```python
from build123d import *

# Parameters (mm, degrees)
AUFSATZ_LINEAR_AUSTRAGEN1_DEPTH    = 5
F_4_0_4_DURCHMESSER_BOHRUNG1_D     = 4
F_4_0_4_DURCHMESSER_BOHRUNG1_DEPTH = 5
F_4_0_4_DURCHMESSER_BOHRUNG1_TIP   = 1.201721238


with BuildPart() as part:
    # Skizze2 → Aufsatz-Linear austragen1 (new body)
    with BuildSketch(Plane.XY):
        with BuildLine():
            Line((1.443375673, 0), (38.556624327, 0))
            ThreePointArc((38.556624327, 0), (39.806624327, -0.334936491), (40.721687836, -1.25))
            Line((40.721687836, -1.25), (50.680145631, -18.498554865))
            ThreePointArc((50.680145631, -18.498554865), (52.51027265, -20.328681884), (55.01027265, -20.998554865))
            Line((55.01027265, -20.998554865), (62.123521304, -20.998554865))
            ThreePointArc((62.123521304, -20.998554865), (64.623521304, -22.034088771), (67.123521304, -20.998554865))
            Line((67.123521304, -20.998554865), (74.793302349, -20.998554865))
            ThreePointArc((74.793302349, -20.998554865), (76.005598743, -20.827762698), (77.123521304, -20.328681884))
            Line((77.123521304, -20.328681884), (77.123521304, -32.998554865))
            ThreePointArc((77.123521304, -32.998554865), (20.139660848, -90.963323142), (-37.5, -33.650635095))
            Line((-37.5, -33.650635095), (-37.501029815, -20.980635095))
            ThreePointArc((-37.501029815, -20.980635095), (-36.382703591, -21.479811555), (-35.17, -21.650635095))
            Line((-35.17, -21.650635095), (-27.5, -21.650635095))
            ThreePointArc((-27.5, -21.650635095), (-25, -22.686169001), (-22.5, -21.650635095))
            Line((-22.5, -21.650635095), (-15.386751346, -21.650635095))
            ThreePointArc((-15.386751346, -21.650635095), (-12.886751346, -20.980762114), (-11.056624327, -19.150635095))
            Line((-11.056624327, -19.150635095), (-0.721687836, -1.25))
            ThreePointArc((-0.721687836, -1.25), (0.193375673, -0.334936491), (1.443375673, 0))
        make_face()
    extrude(amount=AUFSATZ_LINEAR_AUSTRAGEN1_DEPTH)

    # Ø4.0 (4) Durchmesser Bohrung1
    with Locations(Plane.XY.offset(5)):
        with Locations((20, -11.330104149)):
            Hole(F_4_0_4_DURCHMESSER_BOHRUNG1_D / 2, depth=F_4_0_4_DURCHMESSER_BOHRUNG1_DEPTH)
            with Locations((0, 0, -(F_4_0_4_DURCHMESSER_BOHRUNG1_DEPTH + F_4_0_4_DURCHMESSER_BOHRUNG1_TIP / 2))):  # 118° drill point
                Cone(0, F_4_0_4_DURCHMESSER_BOHRUNG1_D / 2, F_4_0_4_DURCHMESSER_BOHRUNG1_TIP, mode=Mode.SUBTRACT)


solid = part.part
```
Can you work these out from the model? Positions are in its coordinate system, mm. A direction names the side the tool comes from. Give positions to 0.01 mm unless a question says otherwise; leave off trailing zeros. Loops run counter-clockwise (first coordinate to the right, second up) from the corner with the lowest first, then second, coordinate; pieces in that order, holes last. Notation, with made-up numbers: M -31,-33.75 L 11,-33.75 A28 cw 11,2.25 Z; hole C 47,-39 d3. An arc over 180 degrees is marked long. One line per question, with ' | ' between items. Start each with the question number.
Q1. If I drill on line 1 (Y direction, x = 20, z = 2.8); line 2 (X direction, y = -66, z = 1.2); line 3 (X direction, y = -10.5, z = 0.5), over which ranges is the centre line in solid material (lowest first)? Write a range as from..to.
Q2. If we mould it in two halves opening along X, with no side actions, what happens to faces 1 (the cylindrical face through (-12.92, -21, 2.46)), 2 (the flat face through (-5.962, -10.326, 2.465)), 3 (the flat face through (21, -45, 5))? For each: +X half, -X half, draft (parallel to the pull), parting line (faces both ways), or undercut.
Q3. For pin 1 Ø1.5 at (x, z) = (59, 3) entering from +Y; pin 2 Ø2.5 at (y, z) = (-29, 2.5) entering from +X; pin 3 Ø2.5 at (x, z) = (-32, 1.5) entering from +Y, each with a flat end and sliding along its axis, tell me the tip position at first contact or that it passes through.
Q4. For faces 4 (the flat face through (-31, -21.651, 2)), 5 (the flat face through (77.124, -27, 2)), which set-ups out of +Z, -Z, +X, -X, +Y, -Y let a thin tool reach every point of the face, with its end or its side?
Q5. If we section it at C-C (y = -75): Please give me the cut outline in (x, z).
Q6. If we section it at A-A (x = 20): Please give me the cut outline in (y, z).
Q7. If we section it at D-D (x = -9.5): Please give me the cut outline in (y, z).
Computed:
1) line 1: y = -90.96..-13.33, -9.33..0 | line 2: x = -27.5..67.13 | line 3: x = -6.06..18.18, 21.82..46.06
2) face 1: undercut | face 2: -X half | face 3: draft
3) pin 1: stops at y = -21 | pin 2: stops at x = 77.12 | pin 3: stops at y = -21.65
4) face 4: +Z, -Z, +Y | face 5: +Z, -Z, +X, +Y, -Y
5) outline: M -19.87,0 L 59.5,0 L 59.5,5 L -19.87,5 Z
6) outline: M -90.96,0 L -13.33,0 L -13.33,5 L -90.96,5 Z; M -9.33,0 L 0,0 L 0,5 L -9.33,5 Z
7) outline: M -82.9,0 L -16.45,0 L -16.45,5 L -82.9,5 Z
